Could you check a few things on this model? Use its own coordinates, in mm. A direction names the side the tool comes from. Give positions to 0.01 mm unless a question says otherwise; leave off trailing zeros. Order: outer loops, then holes, each group sorted by start corner. A loop starts at its lowest first (then second) coordinate and runs counter-clockwise, first axis right, second up. Notation, with made-up numbers: (38.5, -5.5) -> (64.5, -5.5) arc R17 cw to (64.5, 10.5) -> close; hole circle Ø9 at (-8, 14.5). An arc over 180 degrees is marked (long way). Write each question's results on one line, items separated by ' | '.
```python
from build123d import *

# Parameters (mm, degrees)
F0_W     = 152.4
F0_H     = 304.8
F1_DEPTH = 6.35
F2_W     = 9.525
F2_H     = 203.2
F3_DEPTH = 25.4


with BuildPart() as f1:
    # F0 (on Top) → F1 (new body)
    with BuildSketch(Plane.XY):
        with Locations((-76.2, 152.4)):
            Rectangle(F0_W, F0_H)
    extrude(amount=F1_DEPTH)

    # F2 (on face) → F3 (cut)
    with BuildSketch(Plane.XY.offset(6.35)):
        with BuildLine():
            ThreePointArc((-119.38, 254), (-124.1425, 258.7625), (-128.905, 254))
            Line((-128.905, 254), (-119.38, 254))
        make_face()
        with Locations((-124.1425, 152.4)):
            Rectangle(F2_W, F2_H)
        with BuildLine():
            Line((-119.38, 50.8), (-128.905, 50.8))
            ThreePointArc((-128.905, 50.8), (-124.1425, 46.0375), (-119.38, 50.8))
        make_face()
        with BuildLine():
            ThreePointArc((-23.495, 254), (-28.2575, 258.7625), (-33.02, 254))
            Line((-33.02, 254), (-23.495, 254))
        make_face()
        with Locations((-28.2575, 152.4)):
            Rectangle(F2_W, F2_H)
        with BuildLine():
            Line((-23.495, 50.8), (-33.02, 50.8))
            ThreePointArc((-33.02, 50.8), (-28.2575, 46.0375), (-23.495, 50.8))
        make_face()
    extrude(amount=-F3_DEPTH, mode=Mode.SUBTRACT)


solid = f1.part
```
Q1. Suppose I cut it at A-A on y = 64. Please give me the cut outline in (x, z) (3 decimals).
Here are the results:
outline: (-152.4, 0) -> (-128.905, 0) -> (-128.905, 6.35) -> (-152.4, 6.35) -> close; (-119.38, 0) -> (-33.02, 0) -> (-33.02, 6.35) -> (-119.38, 6.35) -> close; (-23.495, 0) -> (0, 0) -> (0, 6.35) -> (-23.495, 6.35) -> close
Q2. Suppose I cut it at B-B on z = 5. Please give me the cut outline in (x, y) (1 decimal).
Here are the results:
outline: (-152.4, 0) -> (0, 0) -> (0, 304.8) -> (-152.4, 304.8) -> close; hole (-128.9, 50.8) arc R4.8 ccw to (-119.4, 50.8) -> (-119.4, 254) arc R4.8 ccw to (-128.9, 254) -> close; hole (-33, 50.8) arc R4.8 ccw to (-23.5, 50.8) -> (-23.5, 254) arc R4.8 ccw to (-33, 254) -> close
Q3. Thinking about a two-plate mould opening in Y: for faces 1 (the flat face through (-77, 304.8, 3)), 2 (the flat face through (-77, 155, 6.35)), 3 (the flat face through (-23.495, 151, 3)), which applies, +Y half, -Y half, draft (parallel to the pull), parting line (faces both ways), or undercut?
Here are the results:
face 1: +Y half | face 2: draft | face 3: undercut
Q4. For faces 4 (the cylindrical face through (-124.04, 258.76, 3.22)), 5 (the flat face through (-77, 0, 3)), which set-ups out of +Z, -Z, +X, -X, +Y, -Y let a thin tool reach every point of the face, with its end or its side?
Here are the results:
face 4: +Z, -Z | face 5: +Z, -Z, +X, -X, -Y
Q5. I need wall thicknesses on line 1 along X through (y, z) = (165.5, 4.75) (3 decimals); line 2 along Y through (x, z) = (-31, 1). Which ranges of each line are inside material? Lowest first, please.
Here are the results:
line 1: x = -152.4 to -128.905, -119.38 to -33.02, -23.495 to 0 | line 2: y = 0 to 46.91, 257.89 to 304.8
Q6. I'm going to push a flat-ended pin straight in: pin 1 Ø3 at (y, z) = (189, 1.5) entering from +X. Where does the tip first touch, or does it pass through?
Here are the results:
pin 1: stops at x = 0
